Can you work these out from the model? Positions are in its coordinate system, mm. A direction names the side the tool comes from. Give positions to 0.01 mm unless a question says otherwise; leave off trailing zeros. Loops run counter-clockwise (first coordinate to the right, second up) from the corner with the lowest first, then second, coordinate; pieces in that order, holes last. Notation, with made-up numbers: (35, -6.5) - (79, -6.5) arc R17 cw to (79, 25.5) - close; hole circle Ø10 at (72.25, -37). An arc over 180 degrees is marked (long way). Answer in a Markdown table with one row per item.
from build123d import *

# Parameters (mm, degrees)
SKETCH1_R                = 8
BOSS_EXTRUDE1_DEPTH      = 30
SKETCH2_R                = 20
BOSS_EXTRUDE2_DEPTH      = 5
CHAMFER1_SIZE            = 2
SKETCH3_R                = 2.5
CUT_EXTRUDE1_DEPTH       = 71.887234394
CIRPATTERN1_COUNT        = 4
FILLET1_R                = 3
MIRROR5_COPY_1_SKETCH_R  = 2.5
MIRROR5_COPY_1_DEPTH     = 71.887234394
MIRROR5_COPY_2_SKETCH_R  = 2.5
MIRROR5_COPY_2_DEPTH     = 71.887234394
MIRROR5_COPY_3_SKETCH_R  = 2.5
MIRROR5_COPY_3_DEPTH     = 71.887234394
CHAMFER1_OF_MIRROR5_SIZE = 2
FILLET1_OF_MIRROR5_R     = 3


with BuildPart() as part:
    # Sketch1 → Boss-Extrude1 (new, symmetric)
    with BuildSketch(Plane.XY):
        Circle(SKETCH1_R)
    extrude(amount=BOSS_EXTRUDE1_DEPTH, both=True)

    # Sketch2 → Boss-Extrude2 (add)
    with BuildSketch(Plane.XY.offset(30)):
        Circle(SKETCH2_R)
    boss_extrude2 = extrude(amount=BOSS_EXTRUDE2_DEPTH)

    # Chamfer1
    chamfer1_edges = [part.edges().sort_by_distance(p)[0] for p in [
        (-20, 0, 35),
    ]]
    chamfer(chamfer1_edges, length=CHAMFER1_SIZE)

    # Sketch3 → Cut-Extrude1 (cut, through all)
    with BuildSketch(Plane.XY.offset(35)):
        with Locations((0, 13)):
            Circle(SKETCH3_R)
    cut_extrude1 = extrude(amount=-CUT_EXTRUDE1_DEPTH, mode=Mode.SUBTRACT)

    # CirPattern1: Cut-Extrude1 ×4 about axis
    cirpattern1_axis = Axis((0, 0, 0), (0, 0, 1))
    for i in range(1, CIRPATTERN1_COUNT):
        add(cut_extrude1.rotate(cirpattern1_axis, i * 360 / CIRPATTERN1_COUNT), mode=Mode.SUBTRACT)

    # Fillet1
    fillet1_edges = [part.edges().sort_by_distance(p)[0] for p in [
        (-8, 0, 30),
    ]]
    fillet(fillet1_edges, radius=FILLET1_R)

    # Mirror5: Boss-Extrude2, Cut-Extrude1 across plane
    add(boss_extrude2.mirror(Plane.XY))
    add(cut_extrude1.mirror(Plane.XY), mode=Mode.SUBTRACT)

    # Mirror5 copy 1 sketch → Mirror5 copy 1 (cut, through all)
    with BuildSketch(Plane.YX.offset(35)):
        with Locations((0, -13)):
            Circle(MIRROR5_COPY_1_SKETCH_R)
    extrude(amount=-MIRROR5_COPY_1_DEPTH, mode=Mode.SUBTRACT)

    # Mirror5 copy 2 sketch → Mirror5 copy 2 (cut, through all)
    with BuildSketch(Plane(origin=(0, 0, -35), x_dir=(-1, 0, 0), z_dir=(0, 0, -1))):
        with Locations((0, -13)):
            Circle(MIRROR5_COPY_2_SKETCH_R)
    extrude(amount=-MIRROR5_COPY_2_DEPTH, mode=Mode.SUBTRACT)

    # Mirror5 copy 3 sketch → Mirror5 copy 3 (cut, through all)
    with BuildSketch(Plane(origin=(0, 0, -35), x_dir=(0, -1, 0), z_dir=(0, 0, -1))):
        with Locations((0, -13)):
            Circle(MIRROR5_COPY_3_SKETCH_R)
    extrude(amount=-MIRROR5_COPY_3_DEPTH, mode=Mode.SUBTRACT)

    # Chamfer1 of Mirror5
    chamfer1_of_mirror5_edges = [part.edges().sort_by_distance(p)[0] for p in [
        (-20, 0, -35),
    ]]
    chamfer(chamfer1_of_mirror5_edges, length=CHAMFER1_OF_MIRROR5_SIZE)

    # Fillet1 of Mirror5
    fillet1_of_mirror5_edges = [part.edges().sort_by_distance(p)[0] for p in [
        (-8, 0, -30),
    ]]
    fillet(fillet1_of_mirror5_edges, radius=FILLET1_OF_MIRROR5_R)


solid = part.part
Q1. If I drill on line 1 (Y direction, x = 0, z = 31.75); line 2 (Z direction, x = 17, y = 2.5); line 3 (Y direction, x = 0, z = -33.05), over which ranges is the centre line in solid material (lowest first)? Write a range as [from, to].
Checked values:
| item | result |
|---|---|
| line 1 | y = [-20, -15.5], [-10.5, 10.5], [15.5, 20] |
| line 2 | z = [-35, -30], [30, 35] |
| line 3 | y = [-19.95, -15.5], [-10.5, 10.5], [15.5, 19.95] |
Q2. For pin 1 (1 mm diameter, centred on y = 7, z = 2, fed in from +X); pin 2 (1 mm diameter, centred on x = 0.5, z = 16, fed in from -Y); pin 3 (10 mm diameter, centred on x = -11, z = -10, fed in from -Y); pin 4 (4.5 mm diameter, centred on x = 0, y = -13, fed in from +Z), each with a flat end and sliding along its axis, tell me the tip position at first contact or that it passes through.
Checked values:
| item | result |
|---|---|
| pin 1 | stops at x = 4.66 |
| pin 2 | stops at y = -8 |
| pin 3 | stops at y = -5.29 |
| pin 4 | passes through |
Q3. Imagine slicing it at C-C, the plane z = -9.5. Write out the boundary of the cut face in (x, y).
Checked values:
| item | result |
|---|---|
| outline | circle Ø16 at (0, 0) |
Q4. If we mould it in two halves opening along Y, with no side actions, what happens to faces 1 (the face through (-4.336, -19.524, -31.479)), 2 (the face through (0.54, -10.56, 32.53)), 3 (the face through (9, -9, -30))? For each: released by +Y, released by -Y, zero draft, split by the parting line, or undercut.
Checked values:
| item | result |
|---|---|
| face 1 | split by the parting line |
| face 2 | undercut |
| face 3 | zero draft |
Q5. Imagine slicing it at A-A, the plane x = -14. Count the separate pieces of the cut face and the enclosed holes in it, and give its area (3 significant figures).
Checked values:
| item | result |
|---|---|
| separate pieces | 4 |
| enclosed holes | 0 |
| area | 228 mm² |
Q6. On a 3-axis mill with a long thin cutter (end or side, diameter ignored), from which of +Z, -Z, +X, -X, +Y, -Y can I reach the whole of each face in a straight line? I mean faces 4 (the face through (9, -9, 30)), 5 (the face through (10.56, 0.54, 32.53)). Say none if no direction works.
Checked values:
| item | result |
|---|---|
| face 4 | none |
| face 5 | +Z, -Z |
